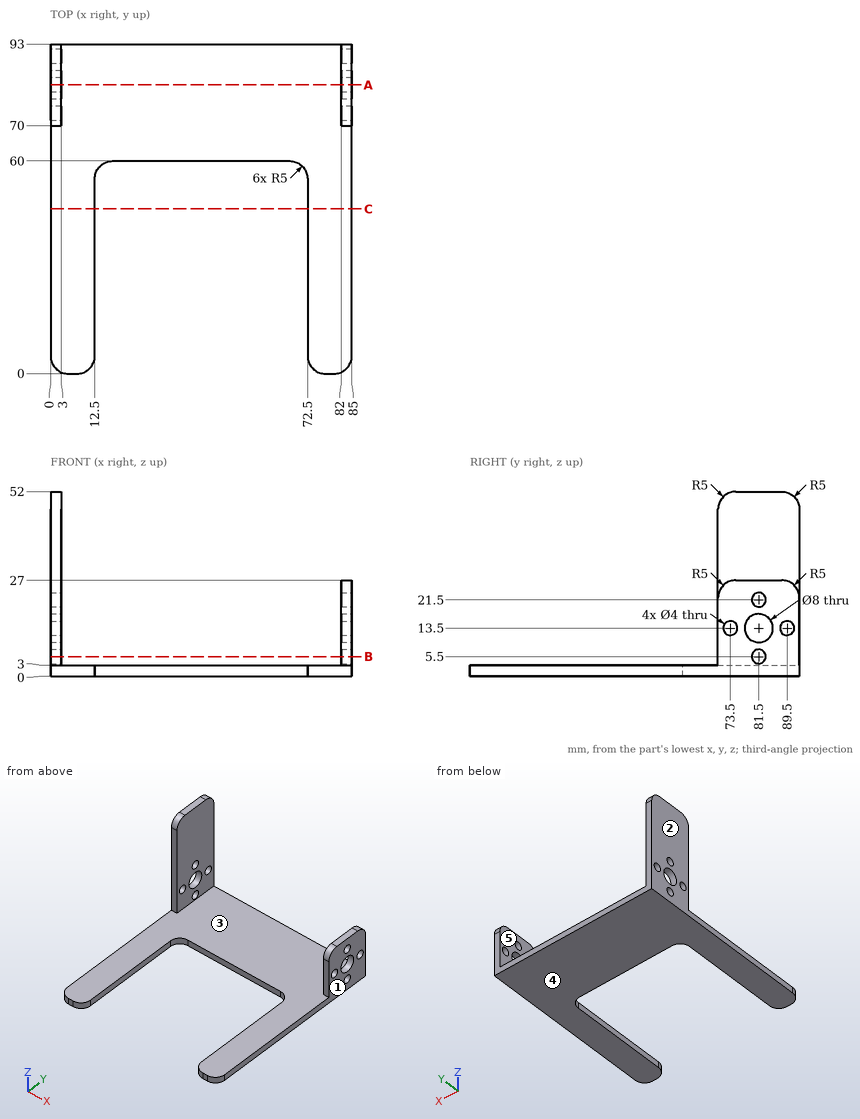
Drawing for the job (mm, zero at the part's lowest x, y, z). A direction names the side the tool comes from. Give positions to 0.01 mm unless a question says otherwise; leave off trailing zeros. Order: outer loops, then holes, each group sorted by start corner. A loop starts at its lowest first (then second) coordinate and runs counter-clockwise, first axis right, second up. Notation, with made-up numbers: M 48,79 L 101,79 A33 ccw 101,109 Z; hole C -38.5,-12.75 d1. An arc over 180 degrees is marked long. Put each result on its own line as item: value. Start each with the question number.
(1) Saw through at C-C, the plane y = 46.5. Write the cut outline in (x, z).
(2) Saw through at B-B, the plane z = 5.5. Write the cut outline in (x, y), then the cut area to 3 significant figures.
(3) Which spindle directions (+Z, -Z, +X, -X, +Y, -Y) get a long thin tool onto all of the face, cutting with end or side? Do the marked faces 4 and 5. Say none if no direction does.
(4) Drill centre lines: line 1 along Z through (x, y) = (2.25, 81.5); line 2 along X through (y, z) = (76.5, 26); line 3 along Z through (x, y) = (64, 81.5). Where is each one in solid material? Low to high.
(5) Saw through at A-A, the plane y = 81.5. Give the number of separate pieces and of enclosed holes in the cut face, then the cut area to 3 significant figures.
(6) Mould opens along X. For the marked faces 1, 2 and 3 say: +X half, -X half, draft (parallel to the pull), parting line (faces both ways), or undercut.
(7) Flat gauge pins, fed straight in: pin 1 Ø5 at (y, z) = (73.5, 13.5) entering from +X; pin 2 Ø3 at (x, y) = (13, 16.5) entering from +Z; pin 3 Ø7 at (y, z) = (81.5, 37) entering from +X; pin 4 Ø2.5 at (x, z) = (53, 2) entering from -Y. Where does each tip first touch, or does it go through?
Check result:
1. outline: M 0,0 L 12.5,0 L 12.5,3 L 0,3 Z; M 72.5,0 L 85,0 L 85,3 L 72.5,3 Z
2. outline: M 0,70 L 3,70 L 3,79.5 L 0,79.5 Z; M 0,83.5 L 3,83.5 L 3,93 L 0,93 Z; M 82,70 L 85,70 L 85,79.5 L 82,79.5 Z; M 82,83.5 L 85,83.5 L 85,93 L 82,93 Z
2. area: 114 mm2
3. face 4: -Z, +X, -X, +Y, -Y
3. face 5: +Z, +Y, -Y
4. line 1: z = 0 to 3.5, 7.5 to 9.5, 17.5 to 19.5, 23.5 to 52
4. line 2: x = 0 to 3, 82 to 85
4. line 3: z = 0 to 3
5. separate pieces: 7
5. enclosed holes: 0
5. area: 378 mm2
6. face 1: +X half
6. face 2: -X half
6. face 3: undercut
7. pin 1: stops at x = 85
7. pin 2: stops at z = 3
7. pin 3: stops at x = 3
7. pin 4: stops at y = 60
